```python
from build123d import *

# Parameters (mm, degrees)
SKETCH1_W           = 1330.706
SKETCH1_H           = 406.4
BOSS_EXTRUDE1_DEPTH = 12.7
SKETCH3_R           = 2.54
SKETCH3_W           = 50.8
SKETCH3_H           = 38.1
SKETCH3_W_2         = 88.9
SKETCH3_W_3         = 17.78
SKETCH3_H_2         = 12.7
SKETCH3_W_4         = 25.4
SKETCH3_W_5         = 39.0906
CUT_EXTRUDE2_DEPTH  = 13.7


with BuildPart() as part:
    # Sketch1 → Boss-Extrude1 (new body)
    with BuildSketch(Plane(origin=(0, 0, 0), x_dir=(1, 0, 0), z_dir=(0, 1, 0))):
        with Locations((665.353, 203.2)):
            Rectangle(SKETCH1_W, SKETCH1_H)
    extrude(amount=BOSS_EXTRUDE1_DEPTH)

    # Sketch3 → Cut-Extrude2 (cut, through all)
    with BuildSketch(Plane.XZ):
        with Locations((89.3953, -278.5618)):
            Circle(SKETCH3_R)
        with Locations((89.3953, -355.6)):
            Circle(SKETCH3_R)
        with Locations((345.3765, -278.5618)):
            Circle(SKETCH3_R)
        with Locations((345.3765, -355.6)):
            Circle(SKETCH3_R)
        with Locations((601.3577, -278.5618)):
            Circle(SKETCH3_R)
        with Locations((601.3577, -355.6)):
            Circle(SKETCH3_R)
        with Locations((729.3483, -278.5618)):
            Circle(SKETCH3_R)
        with Locations((729.3483, -355.6)):
            Circle(SKETCH3_R)
        with Locations((985.3295, -278.5618)):
            Circle(SKETCH3_R)
        with Locations((985.3295, -355.6)):
            Circle(SKETCH3_R)
        with Locations((1241.3107, -278.5618)):
            Circle(SKETCH3_R)
        with Locations((1241.3107, -355.6)):
            Circle(SKETCH3_R)
        with Locations((57.15, -318.77)):
            Rectangle(SKETCH3_W, SKETCH3_H)
        with Locations((294.0812, -318.77)):
            Rectangle(SKETCH3_W_2, SKETCH3_H)
        with Locations((166.0906, -318.77)):
            Rectangle(SKETCH3_W_2, SKETCH3_H)
        with Locations((35.56, -361.95)):
            Rectangle(SKETCH3_W_3, SKETCH3_H_2)
        with Locations((422.0718, -318.77)):
            Rectangle(SKETCH3_W_2, SKETCH3_H)
        with Locations((550.0624, -318.77)):
            Rectangle(SKETCH3_W_2, SKETCH3_H)
        with Locations((678.053, -318.77)):
            Rectangle(SKETCH3_W_2, SKETCH3_H)
        with Locations((806.0436, -318.77)):
            Rectangle(SKETCH3_W_2, SKETCH3_H)
        with Locations((934.0342, -318.77)):
            Rectangle(SKETCH3_W_2, SKETCH3_H)
        with Locations((1062.0248, -318.77)):
            Rectangle(SKETCH3_W_2, SKETCH3_H)
        with Locations((1190.0154, -318.77)):
            Rectangle(SKETCH3_W_2, SKETCH3_H)
        with Locations((1286.256, -318.77)):
            Rectangle(SKETCH3_W_4, SKETCH3_H)
        with Locations((408.8765, -273.05)):
            Rectangle(SKETCH3_W_5, SKETCH3_H_2)
        with Locations((35.56, -273.05)):
            Rectangle(SKETCH3_W_3, SKETCH3_H_2)
        with Locations((152.8953, -273.05)):
            Rectangle(SKETCH3_W_5, SKETCH3_H_2)
        with Locations((152.8953, -361.95)):
            Rectangle(SKETCH3_W_5, SKETCH3_H_2)
        with Locations((280.8859, -273.05)):
            Rectangle(SKETCH3_W_5, SKETCH3_H_2)
        with Locations((280.8859, -361.95)):
            Rectangle(SKETCH3_W_5, SKETCH3_H_2)
        with Locations((408.8765, -361.95)):
            Rectangle(SKETCH3_W_5, SKETCH3_H_2)
        with Locations((536.8671, -361.95)):
            Rectangle(SKETCH3_W_5, SKETCH3_H_2)
        with Locations((536.8671, -273.05)):
            Rectangle(SKETCH3_W_5, SKETCH3_H_2)
        with Locations((664.8577, -361.95)):
            Rectangle(SKETCH3_W_5, SKETCH3_H_2)
        with Locations((664.8577, -273.05)):
            Rectangle(SKETCH3_W_5, SKETCH3_H_2)
        with Locations((792.8483, -273.05)):
            Rectangle(SKETCH3_W_5, SKETCH3_H_2)
        with Locations((920.8389, -361.95)):
            Rectangle(SKETCH3_W_5, SKETCH3_H_2)
        with Locations((792.8483, -361.95)):
            Rectangle(SKETCH3_W_5, SKETCH3_H_2)
        with Locations((920.8389, -273.05)):
            Rectangle(SKETCH3_W_5, SKETCH3_H_2)
        with Locations((1048.8295, -361.95)):
            Rectangle(SKETCH3_W_5, SKETCH3_H_2)
        with Locations((1048.8295, -273.05)):
            Rectangle(SKETCH3_W_5, SKETCH3_H_2)
        with Locations((1176.8201, -273.05)):
            Rectangle(SKETCH3_W_5, SKETCH3_H_2)
        with Locations((1176.8201, -361.95)):
            Rectangle(SKETCH3_W_5, SKETCH3_H_2)
        with Locations((1294.1554, -361.95)):
            Rectangle(SKETCH3_W_3, SKETCH3_H_2)
        with Locations((1294.1554, -273.05)):
            Rectangle(SKETCH3_W_3, SKETCH3_H_2)
    extrude(amount=-CUT_EXTRUDE2_DEPTH, mode=Mode.SUBTRACT)


solid = part.part
```
The model under review builds one solid part; all positions refer to its coordinate system, in mm. Round coordinates to 2 decimals unless told otherwise and drop trailing zeros. Loops run counter-clockwise (first coordinate to the right, second up) from the corner with the lowest first, then second, coordinate; pieces in that order, holes last.
1) Clearance check with a flat-ended pin moving along its axis: P1, Ø6.5, axis at y = 8, z = -316, coming from the -X side. State where the tip first meets the part, or that it passes through.
Values follow:
P1: stops at x = 0
2) Wall thickness on line 1 along Z through (x, y) = (527, 1); line 2 along Z through (x, y) = (716, 10.5): over which ranges is each line inside the solid? List them lowest first.
Values follow:
line 1: z = -406.4 to -368.3, -355.6 to -337.82, -299.72 to -279.4, -266.7 to 0
line 2: z = -406.4 to -337.82, -299.72 to 0
3) Consider section B-B on y = 6.5. Give the number of separate pieces and of enclosed holes in the cut face, then the cut area to 3 significant figures.
Values follow:
separate pieces: 1
enclosed holes: 45
area: 497,000 mm2
4) Consider section A-A on x = 287. State the section outline as (y, z) points.
Values follow:
outline: (0, -406.4) - (12.7, -406.4) - (12.7, -368.3) - (0, -368.3) - close; (0, -355.6) - (12.7, -355.6) - (12.7, -337.82) - (0, -337.82) - close; (0, -299.72) - (12.7, -299.72) - (12.7, -279.4) - (0, -279.4) - close; (0, -266.7) - (12.7, -266.7) - (12.7, 0) - (0, 0) - close
